```python
from build123d import *

# Parameters (mm, degrees)
SKETCH8_R          = 19.05
CUT_EXTRUDE2_DEPTH = 115.123474798
SKETCH9_R          = 6.35
CUT_EXTRUDE3_DEPTH = 106.875658203
CIRPATTERN1_COUNT  = 4
FILLET1_R          = 6.35
CHAMFER1_SIZE      = 2.032


with BuildPart() as part:
    # Sketch7 → Revolve1 (revolve)
    with BuildSketch(Plane.XY, mode=Mode.PRIVATE) as revolve1_sk:
        Polygon((34.925, 0), (69.85, 0), (69.85, -19.05), (0, -19.05), (0, 0), (0, 38.1), (34.925, 38.1), align=None)
    revolve(revolve1_sk.sketch.rotate(Axis((0, 38.1, 0), (0, -1, 0)), 270), axis=Axis((0, 38.1, 0), (0, -1, 0)))

    # Sketch8 → Cut-Extrude2 (cut, through all)
    with BuildSketch(Plane(origin=(0, 38.1, 0), x_dir=(1, 0, 0), z_dir=(0, 1, 0))):
        with Locations(Location((0, 0, 0), (0, 0, 270))):
            Circle(SKETCH8_R)
    extrude(amount=-CUT_EXTRUDE2_DEPTH, mode=Mode.SUBTRACT)

    # Sketch9 → Cut-Extrude3 (cut, through all)
    with BuildSketch(Plane(origin=(0, 0, 0), x_dir=(1, 0, 0), z_dir=(0, 1, 0))):
        with Locations(Location((0, 53.975, 0), (0, 0, 270))):
            Circle(SKETCH9_R)
    cut_extrude3 = extrude(amount=-CUT_EXTRUDE3_DEPTH, mode=Mode.SUBTRACT)

    # CirPattern1: Cut-Extrude3 ×4 about axis
    cirpattern1_axis = Axis((0, 0, 0), (0, 1, 0))
    for i in range(1, CIRPATTERN1_COUNT):
        add(cut_extrude3.rotate(cirpattern1_axis, i * 360 / CIRPATTERN1_COUNT), mode=Mode.SUBTRACT)

    # Fillet1
    fillet1_edges = [part.edges().sort_by_distance(p)[0] for p in [
        (0, 38.1, 34.925),
        (0, 0, 34.925),
        (0, 0, 69.85),
    ]]
    fillet(fillet1_edges, radius=FILLET1_R)

    # Chamfer1
    chamfer1_edges = [part.edges().sort_by_distance(p)[0] for p in [
        (0, 38.1, -19.05),
    ]]
    chamfer(chamfer1_edges, length=CHAMFER1_SIZE)


solid = part.part
```
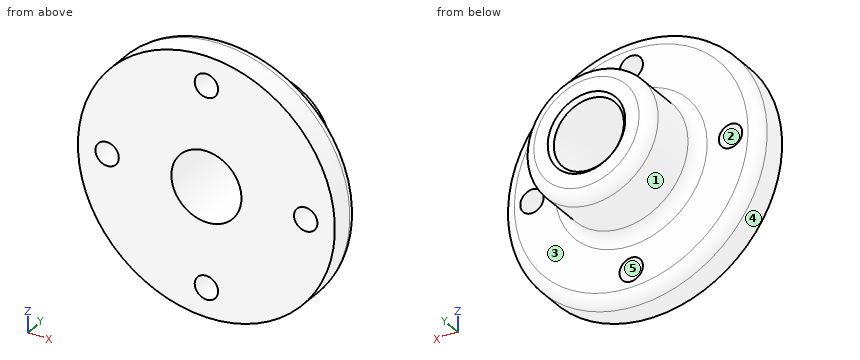
Work out the finished part from the listing and answer in its coordinate system (mm). Face numbers are marked on the shaded views. A direction names the side the tool comes from. Give positions to 0.01 mm unless a question says otherwise; leave off trailing zeros. Write each loop counter-clockwise with the first axis right and the second up, starting at its lowest first coordinate (ties: lowest second). Pieces come first, ordered by that corner, then holes.
(1) The part is cut by section C-C on y = 26. Write down the section's boundary in (x, z) (3 decimals).
Final values:
outline: circle Ø69.85 at (0, 0); hole circle Ø38.1 at (0, 0)
(2) The part is cut by section A-A on x = 0. Write down the section's boundary in (y, z) (3 decimals).
Final values:
outline: (-19.05, -69.85) - (-6.35, -69.85) arc R6.35 ccw to (0, -63.5) - (0, -60.325) - (-19.05, -60.325) - close; (-19.05, -47.625) - (0, -47.625) - (0, -41.275) arc R6.35 cw to (6.35, -34.925) - (31.75, -34.925) arc R6.35 ccw to (38.1, -28.575) - (38.1, -21.082) - (36.068, -19.05) - (-19.05, -19.05) - close; (-19.05, 19.05) - (36.068, 19.05) - (38.1, 21.082) - (38.1, 28.575) arc R6.35 ccw to (31.75, 34.925) - (6.35, 34.925) arc R6.35 cw to (0, 41.275) - (0, 47.625) - (-19.05, 47.625) - close; (-19.05, 60.325) - (0, 60.325) - (0, 63.5) arc R6.35 ccw to (-6.35, 69.85) - (-19.05, 69.85) - close
(3) The mould has two halves that part along X. Classify the marked faces 3, 4 and 5: pulls with the +X half, pulls with the -X half, needs draft (parallel to the pull), parting line crosses it, or undercut.
Final values:
face 3: needs draft
face 4: parting line crosses it
face 5: undercut
(4) The part is cut by section B-B on z = 0. Write down the section's boundary in (x, y) (3 decimals), plus the area to 3 significant figures.
Final values:
outline: (-69.85, -19.05) - (-60.325, -19.05) - (-60.325, 0) - (-63.5, 0) arc R6.35 ccw to (-69.85, -6.35) - close; (-47.625, -19.05) - (-19.05, -19.05) - (-19.05, 36.068) - (-21.082, 38.1) - (-28.575, 38.1) arc R6.35 ccw to (-34.925, 31.75) - (-34.925, 6.35) arc R6.35 cw to (-41.275, 0) - (-47.625, 0) - close; (19.05, -19.05) - (47.625, -19.05) - (47.625, 0) - (41.275, 0) arc R6.35 cw to (34.925, 6.35) - (34.925, 31.75) arc R6.35 ccw to (28.575, 38.1) - (21.082, 38.1) - (19.05, 36.068) - close; (60.325, -19.05) - (69.85, -19.05) - (69.85, -6.35) arc R6.35 ccw to (63.5, 0) - (60.325, 0) - close
area: 2,640 mm2
(5) Which of the six approach directions +Z, -Z, +X, -X, +Y, -Y give full straight-line access (tool end or side, diameter ignored) to the marked faces 1 and 2?
Final values:
face 1: +Y
face 2: +Y, -Y
(6) Straight lines are drawn through the part: line 1 (X direction, y = 14.5, z = 1); line 2 (X direction, y = -4, z = 4.5); line 3 (X direction, y = 10, z = 17). For each, find the intervals that lie inside material, in ascending order.
Final values:
line 1: x = -34.91 to -19.02, 19.02 to 34.91
line 2: x = -69.25 to -58.46, -49.49 to -18.51, 18.51 to 49.49, 58.46 to 69.25
line 3: x = -30.51 to -8.6, 8.6 to 30.51
(7) Flat-ended cylindrical pins translate along their axes: pin 1 Ø10 at (x, z) = (0, -53.975) entering from +Y; pin 2 Ø4 at (y, z) = (-4.5, 38) entering from +X; pin 3 Ø3 at (x, z) = (35, -20) entering from +Y; pin 4 Ø10 at (y, z) = (-6.5, -36.5) entering from +X. Find the tip coordinate at first contact, or state that the pin passes through.
Final values:
pin 1: passes through
pin 2: stops at x = 59.66
pin 3: stops at y = 0.5
pin 4: stops at x = 62.34
